Source: CAD feature listing. Evaluate the final solid. Frame: model axes, mm. Face numbers are marked on the shaded views. A direction names the side the tool comes from. Coordinates: 2 decimals unless noted, no trailing zeros. Write each loop counter-clockwise with the first axis right and the second up, starting at its lowest first coordinate (ties: lowest second). Pieces come first, ordered by that corner, then holes. Notation, with made-up numbers: M 22,-13.5 L 74,-13.5 A20 cw 74,10.5 Z; hole C -38.5,18.5 d10. An arc over 180 degrees is marked long. One line per item, written item: value. Start each with the question number.
Item 1: Set-up query: the marked faces 4, 5 and 6. Return all of +Z, -Z, +X, -X, +Y, -Y with unobstructed straight access to the full face (end or side cutting, diameter ignored); none if empty.
Item 2: Cut plane A-A, the plane z = -23.5. Output: boundary loops of the cut face in (x, y).
Item 3: Cut plane C-C, the plane y = 43. Output: boundary loops of the cut face in (x, z).
Item 4: Ray query, L1, parallel to X at y = 0.1, z = -36; L2, parallel to Z at x = 2.5, y = 29.5; L3, parallel to Y at x = 5, z = -22. Return the intervals inside material, ascending. Write a range as from..to.
Item 5: Cut plane D-D, the plane z = -36. Output: boundary loops of the cut face in (x, y), then the cut area to 3 significant figures.
Item 6: Pin query (flat end, axial travel): P1, Ø4, axis at x = 6.5, z = -20, coming from the -Y side; P2, Ø5, axis at x = 8, y = 11.5, coming from the -Z side; P3, Ø1.5, axis at x = 7, y = 13, coming from the -Z side. Return the tip coordinate at first contact, or that it passes through.
Item 7: Mould query, pull axis Z, two halves, no side actions, for the marked faces 1, 2 and 3. Classes: released by +Z, released by -Z, zero draft, split by the parting line, or undercut.
Item 8: Cut plane B-B, the plane x = 11.5. Output: boundary loops of the cut face in (y, z).
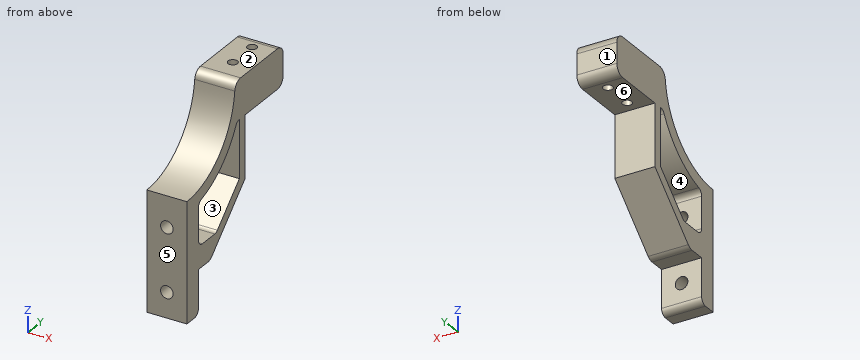
```python
from build123d import *

# Parameters (mm, degrees)
BOSS_EXTRUDE2_DEPTH   = 12.7
CROQUIS3_R            = 2
CORTAR_EXTRUIR2_DEPTH = 25
CROQUIS5_R            = 1.5
CORTAR_EXTRUIR3_DEPTH = 17


with BuildPart() as part:
    # Sketch1 → Boss-Extrude2 (new body)
    with BuildSketch(Plane(origin=(0, 0, 0), x_dir=(0, 0, -1), z_dir=(1, 0, 0))):
        with BuildLine():
            Line((49.204101374, 10.956842444), (33.23486306, 28.251581588))
            Line((33.23486306, 28.251581588), (13.61439919, 28.251581588))
            Line((13.61439919, 28.251581588), (13.61439919, 39.964229912))
            Line((13.61439919, 39.964229912), (13.61439919, 45))
            ThreePointArc((13.61439919, 45), (12.735719533, 47.121320344), (10.61439919, 48))
            Line((10.61439919, 48), (4.084684606, 48))
            ThreePointArc((4.084684606, 48), (1.963364263, 47.121320344), (1.084684606, 45))
            Line((1.084684606, 45), (1.084684606, 25.857413306))
            ThreePointArc((1.084684606, 25.857413306), (1.858719017, 23.846175579), (3.781402736, 22.872782658))
            ThreePointArc((3.781402736, 22.872782658), (19.803767064, 14.76117498), (26.254053819, -1.999139412))
            Line((26.254053819, -1.999139412), (64, -1.999139412))
            Line((64, -1.999139412), (64, 2.000860588))
            ThreePointArc((64, 2.000860588), (63.414213562, 3.41507415), (62, 4.000860588))
            Line((62, 4.000860588), (50, 4.000860588))
            Line((50, 4.000860588), (50, 8.921667481))
            ThreePointArc((50, 8.921667481), (49.793949187, 10.014300969), (49.204101374, 10.956842444))
        make_face()
        with BuildLine():
            Line((42.469400916, 13.828321623), (31.921640745, 25.251581588))
            Line((31.921640745, 25.251581588), (13.61439919, 25.251581588))
            ThreePointArc((13.61439919, 25.251581588), (13.901973758, 24.218334695), (14.681998331, 23.482223332))
            ThreePointArc((14.681998331, 23.482223332), (23.753909667, 15.98324163), (29.068629616, 5.481429706))
            ThreePointArc((29.068629616, 5.481429706), (29.78321361, 4.413589067), (31, 4.000860588))
            Line((31, 4.000860588), (41, 4.000860588))
            ThreePointArc((41, 4.000860588), (42.414213562, 4.586647025), (43, 6.000860588))
            Line((43, 6.000860588), (43, 12.471538314))
            ThreePointArc((43, 12.471538314), (42.862632792, 13.199960639), (42.469400916, 13.828321623))
        make_face(mode=Mode.SUBTRACT)
    extrude(amount=BOSS_EXTRUDE2_DEPTH)

    # Croquis3 → Cortar-Extruir2 (cut)
    with BuildSketch(Plane(origin=(0, 4.000860588, 0), x_dir=(1, 0, 0), z_dir=(0, 1, 0))):
        with Locations(Location((6.35, 56, 0), (0, 0, 270))):
            Circle(CROQUIS3_R)
        with Locations(Location((6.35, 36, 0), (0, 0, 270))):
            Circle(CROQUIS3_R)
    extrude(amount=-CORTAR_EXTRUIR2_DEPTH, mode=Mode.SUBTRACT)

    # Croquis5 → Cortar-Extruir3 (cut)
    with BuildSketch(Plane(origin=(0, 0, -13.61439919), x_dir=(-1, 0, 0), z_dir=(0, 0, -1))):
        with Locations(Location((-6.35, 32.251581588, 0), (0, 0, 90))):
            Circle(CROQUIS5_R)
        with Locations(Location((-6.35, 42.251581588, 0), (0, 0, 90))):
            Circle(CROQUIS5_R)
    extrude(amount=-CORTAR_EXTRUIR3_DEPTH, mode=Mode.SUBTRACT)


solid = part.part
```
From the geometry:
1. face 4: +X, -X
1. face 5: +Z, -Z, +X, -X, -Y
1. face 6: -Z, +X, -X, +Y
2. outline: M 0,9.41 L 12.7,9.41 L 12.7,16.3 L 0,16.3 Z; M 0,25.25 L 12.7,25.25 L 12.7,28.25 L 0,28.25 Z
3. outline: M 0,-13.61 L 5.05,-13.61 L 5.05,-1.08 L 0,-1.08 Z; M 7.65,-13.61 L 12.7,-13.61 L 12.7,-1.08 L 7.65,-1.08 Z
4. L1: x = 0..4.35, 8.35..12.7
4. L2: z = -13.61..-1.08
4. L3: y = 11.95..17.98, 25.25..28.25
5. outline: M 0,-2 L 4.35,-2 L 4.35,4 L 0,4 Z; M 0,20.83 L 12.7,20.83 L 12.7,25.26 L 0,25.26 Z; M 8.35,-2 L 12.7,-2 L 12.7,4 L 8.35,4 Z
5. area: 108 mm²
6. P1: stops at y = 11.95
6. P2: stops at z = -50
6. P3: stops at z = -48.01
7. face 1: zero draft
7. face 2: released by +Z
7. face 3: undercut
8. outline: M -2,-64 L 2,-64 A2 ccw 4,-62 L 4,-50 L 8.92,-50 A3 ccw 10.96,-49.2 L 28.25,-33.23 L 28.25,-13.61 L 45,-13.61 A3 ccw 48,-10.61 L 48,-4.08 A3 ccw 45,-1.08 L 25.86,-1.08 A3 ccw 22.87,-3.78 A25 cw -2,-26.25 Z; hole M 4,-41 A2 ccw 6,-43 L 12.47,-43 A2 ccw 13.83,-42.47 L 25.25,-31.92 L 25.25,-13.61 A2 ccw 23.48,-14.68 A28.8 cw 5.48,-29.07 A2 ccw 4,-31 Z
